For this review, use the dimensioned drawing (mm, ordinates from the lowest corner) and the shaded views. Give positions to 0.01 mm unless a question says otherwise; leave off trailing zeros. Loops run counter-clockwise (first coordinate to the right, second up) from the corner with the lowest first, then second, coordinate; pieces in that order, holes last. Notation, with made-up numbers: (53.5, 39.5) - (59.5, 39.5) arc R25 ccw to (59.5, 58.5) - close; hole circle Ø7 at (68, 48). An arc over 180 degrees is marked (long way). Put each result on its own line as item: value.
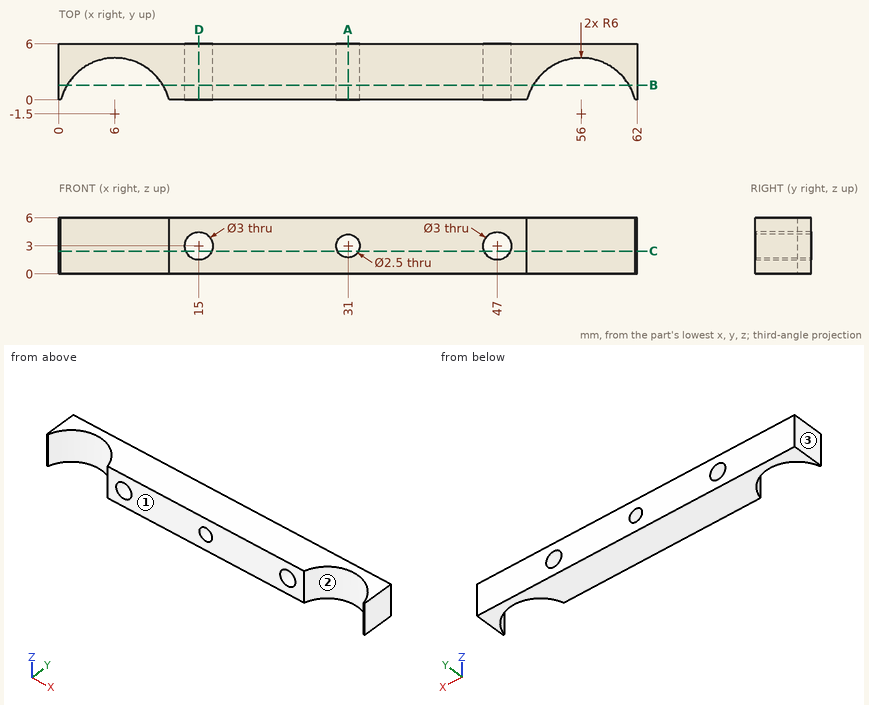
1) Draft analysis for pull direction X (two halves, no side actions). For the marked faces 1, 2 and 3, state which applies: pulls with the +X half, pulls with the -X half, needs draft (parallel to the pull), parting line crosses it, or undercut.
Geometry check:
face 1: needs draft
face 2: undercut
face 3: pulls with the -X half
2) Take a section at B-B on y = 1.6. State the section outline as (x, z) points.
Geometry check:
outline: (0, 0) - (0.86, 0) - (0.86, 6) - (0, 6) - close; (11.14, 0) - (50.86, 0) - (50.86, 6) - (11.14, 6) - close; (61.14, 0) - (62, 0) - (62, 6) - (61.14, 6) - close; hole circle Ø3 at (15, 3); hole circle Ø2.5 at (31, 3); hole circle Ø3 at (47, 3)
3) Take a section at D-D on x = 15. State the section outline as (y, z) points.
Geometry check:
outline: (0, 0) - (6, 0) - (6, 1.5) - (0, 1.5) - close; (0, 4.5) - (6, 4.5) - (6, 6) - (0, 6) - close
4) Wall thickness on line 1 (X direction, y = 1.75, z = 3); line 2 (X direction, y = 2.95, z = 5.05); line 3 (X direction, y = 3.2, z = 3): over which ranges is each line inside the solid? List them lowest first.
Geometry check:
line 1: x = 0 to 0.96, 11.04 to 13.5, 16.5 to 29.75, 32.25 to 45.5, 48.5 to 50.96, 61.04 to 62
line 2: x = 0 to 1.98, 10.02 to 51.98, 60.02 to 62
line 3: x = 0 to 2.27, 9.73 to 13.5, 16.5 to 29.75, 32.25 to 45.5, 48.5 to 52.27, 59.73 to 62
5) Take a section at C-C on z = 2.45. State the section outline as (x, y) points.
Geometry check:
outline: (0, 0) - (0.19, 0) arc R6 cw to (11.81, 0) - (13.6, 0) - (13.6, 6) - (0, 6) - close; (16.4, 0) - (29.88, 0) - (29.88, 6) - (16.4, 6) - close; (32.12, 0) - (45.6, 0) - (45.6, 6) - (32.12, 6) - close; (48.4, 0) - (50.19, 0) arc R6 cw to (61.81, 0) - (62, 0) - (62, 6) - (48.4, 6) - close
6) Take a section at A-A on x = 31. State the section outline as (y, z) points.
Geometry check:
outline: (0, 0) - (6, 0) - (6, 1.75) - (0, 1.75) - close; (0, 4.25) - (6, 4.25) - (6, 6) - (0, 6) - close
